Autodesk Inventor part; units mm, degrees
ref_plane "YZ Plane" through (0, 0, 0) normal (1, 0, 0) x (0, 1, 0)
ref_plane "XZ Plane" through (0, 0, 0) normal (0, 1, 0) x (-1, 0, 0)
ref_plane "XY Plane" through (0, 0, 0) normal (0, 0, 1) x (1, 0, 0)
sketch "Sketch1" plane through (0, 0, 0) normal (0, 1, 0) x (-1, 0, 0)
  line L0 (0, 0) -> (30, 0)
  line L1 (30, 0) -> (30, 100)
  line L2 (30, 100) -> (0, 100)
  line L3 (0, 100) -> (0, 0)
  circle A0 centre (20, 90) radius 0.75
  circle A1 centre (20, 10) radius 0.75
  line L4 (3, 97) -> (3, 3)
  line L5 (30, 100) -> (16, 100)
  line L6 (16, 100) -> (16, 91)
  line L7 (21, 86) -> (30, 86)
  line L8 (30, 86) -> (30, 100)
  line L9 (30, 0) -> (16, 0)
  line L10 (16, 0) -> (16, 9)
  line L11 (21, 14) -> (30, 14)
  line L12 (30, 14) -> (30, 0)
  line L13 (27, 86) -> (27, 14)
  line L14 (3, 97) -> (16, 97)
  line L15 (3, 3) -> (16, 3)
  arc A2 (16, 91) -> (21, 86) centre (21, 91) ccw
  arc A3 (21, 14) -> (16, 9) centre (21, 9) ccw
  point P0 (16, 86)
  point P1 (16, 14)
  dimension "d0" = 30
  dimension "d1" = 100
  dimension "d4" = 94
  dimension "d5" = 14
  dimension "d6" = 14
  dimension "d7" = 14
  dimension "d10" = 5
extrude "Extrusion1" add sketch "Sketch1" along normal blind 2 contours L3 L2 L6 L14 L4 L15 L10 L0 | L10 A3 L11 L1 L0 | L2 L1 L7 A2 L6 | L11 L13 L7 L1
sketch "Sketch2" plane through (0, 2, 0) normal (0, 1, 0) x (1, 0, 0)
  line L0 (-30, 0) -> (-30, -100)
  line L1 (-30, -30) -> (-180, -30)
  line L2 (-180, -30) -> (-180, -70)
  line L3 (-180, -70) -> (-30, -70)
  line L4 (-30, -35) -> (-160, -35)
  line L5 (-160, -35) -> (-160, -65)
  line L6 (-160, -65) -> (-30, -65)
  circle A0 centre (-170, -38) radius 1.5
  circle A1 centre (-170, -62) radius 1.5
  point P0 (0, 0)
  point P1 (-180, -38)
  point P2 (-180, -62)
  point P3 (-180, -62)
  dimension "d11" = 130
  dimension "d12" = 30
  dimension "d13" = 3
  dimension "d14" = 3
extrude "Extrusion2" add sketch "Sketch2" along normal blind 2 from surface at -2 contours L0 L4 L5 L6 L3 L2 L1
sketch "Sketch5" plane through (0, 2, 0) normal (0, 1, 0) x (1, 0, 0)
  point P0 (0, 0)
properties part number "druga czesc"
Verification items for the finished model (mm, model axes). A direction names the side the tool comes from. Give positions to 0.01 mm unless a question says otherwise; leave off trailing zeros. Write each loop counter-clockwise with the first axis right and the second up, starting at its lowest first coordinate (ties: lowest second). Pieces come first, ordered by that corner, then holes. Notation, with made-up numbers: M -18,-17 L -4,-17 A27 cw -4,22 Z; hole C 4.5,-32 d7. An arc over 180 degrees is marked long. Write item = value, one per line.
(1) Sectioned sample at C-C (z = 49). Record the cut outline in (x, y).
Found:
outline = M -180,0 L -160,0 L -160,2 L -180,2 Z; M -30,0 L -27,0 L -27,2 L -30,2 Z; M -3,0 L 0,0 L 0,2 L -3,2 Z
(2) Draft check along X on faces 1 (the face through (-83, 2, 69)), 2 (the face through (-18, 1, 87)). Enter one of: released by +X, released by -X, zero draft, split by the parting line, or undercut.
Found:
face_1 = zero draft
face_2 = undercut
(3) Sectioned sample at B-B (x = -71). Record the cut outline in (y, z), then the cut area to 3 significant figures.
Found:
outline = M 0,30 L 2,30 L 2,35 L 0,35 Z; M 0,65 L 2,65 L 2,70 L 0,70 Z
area = 20.0 mm2
(4) Sectioned sample at A-A (z = 24.5). Record the cut outline in (x, y).
Found:
outline = M -30,0 L -27,0 L -27,2 L -30,2 Z; M -3,0 L 0,0 L 0,2 L -3,2 Z
(5) Access from +Z, -Z, +X, -X, +Y, -Y to the whole of each face (thin tool, end or side, straight path). Record for faces 3 (the face through (-17, 1, 12)), 4 (the face through (-83, 0, 69)).
Found:
face_3 = +Y, -Y
face_4 = +Z, -Z, +X, -X, -Y
(6) Material ranges on line 1 (X direction, y = 0.8, z = 62); line 2 (X direction, y = 1.3, z = 44); line 3 (Z direction, x = -170, y = 1.5), recorded low to high.
Found:
line_1 = -180 to -171.5, -168.5 to -160, -30 to -27, -3 to 0
line_2 = -180 to -160, -30 to -27, -3 to 0
line_3 = 30 to 36.5, 39.5 to 60.5, 63.5 to 70
(7) Go/stop test with flat-tipped pins: pin 1 Ø1 at (x, y) = (-124, 0.5) entering from +Z; pin 2 Ø1.8 at (x, z) = (-170, 62) entering from -Y; pin 3 Ø1 at (y, z) = (1.5, 25.5) entering from -X. Record where each tip stops, or that it passes through.
Found:
pin_1 = 70
pin_2 = through
pin_3 = -30
(8) Sectioned sample at D-D (y = 1.5). Record the cut outline in (x, z).
Found:
outline = M -180,30 L -30,30 L -30,0 L 0,0 L 0,100 L -30,100 L -30,70 L -180,70 Z; hole C -170,38 d3; hole C -170,62 d3; hole M -160,35 L -30,35 L -30,65 L -160,65 Z; hole M -27,14 L -21,14 A5 cw -16,9 L -16,3 L -3,3 L -3,97 L -16,97 L -16,91 A5 cw -21,86 L -27,86 Z; hole C -20,10 d1.5; hole C -20,90 d1.5
